Autodesk Inventor part; units mm, degrees
ref_plane "YZ Plane" through (0, 0, 0) normal (1, 0, 0) x (0, 1, 0)
ref_plane "XZ Plane" through (0, 0, 0) normal (0, 1, 0) x (-1, 0, 0)
ref_plane "XY Plane" through (0, 0, 0) normal (0, 0, 1) x (1, 0, 0)
sketch "Sketch1" plane through (0, 0, 0) normal (0, 0, 1) x (1, 0, 0)
  circle A0 centre (8, -7) radius 1.6
  circle A1 centre (-8, 7) radius 1.6
  circle A2 centre (-2.5, 4.7) radius 0.8
  circle A3 centre (2.5001, 4.7) radius 0.8
  line L0 (-11, 10) -> (-11, -10)
  line L1 (-11, -10) -> (11, -10)
  line L2 (11, -10) -> (11, 10)
  line L3 (11, 10) -> (-11, 10)
  line L4 (-11.2, -10.2) -> (-11.2, 10.2)
  line L5 (-11.2, 10.2) -> (11.2, 10.2)
  line L6 (11.2, 10.2) -> (11.2, -10.2)
  line L7 (11.2, -10.2) -> (-11.2, -10.2)
  circle A4 centre (-8, 7) radius 1.4
  circle A5 centre (8, -7) radius 1.4
  line L8 (-12.2, 11.2) -> (-12.2, -11.2)
  line L9 (-12.2, -11.2) -> (12.2, -11.2)
  line L10 (12.2, -11.2) -> (12.2, 11.2)
  line L11 (12.2, 11.2) -> (-12.2, 11.2)
  circle A6 centre (2.54, -5.9) radius 0.4
  circle A7 centre (-2.54, -5.9) radius 0.4
  circle A8 centre (0, -5.9) radius 0.4
  circle A9 centre (3.5, -7.425) radius 0.5
  circle A10 centre (-3.5, -7.425) radius 0.5
  circle A11 centre (0.6, -3.225) radius 0.3
  circle A12 centre (0.6, -4.425) radius 0.3
  circle A13 centre (-0.6, -3.225) radius 0.3
  circle A14 centre (-0.6, -4.425) radius 0.3
  point P0 (0, 0)
  dimension "d6" = 15
  dimension "d7" = 10
  dimension "d0" = 0.2
  dimension "d1" = 0.2
  dimension "d2" = 0.2
  dimension "d3" = 1
extrude "Extrusion1" add sketch "Sketch1" against normal blind 4 contours A4 | A5 | L11 L10 L9 L8
sketch "Sketch2" plane through (0, 0, -4) normal (0, 0, -1) x (-1, 0, 0)
  line L0 (-12.2, -11.2) -> (12.2, -11.2)
  line L1 (12.2, -11.2) -> (12.2, 11.2)
  line L2 (12.2, 11.2) -> (-12.2, 11.2)
  line L3 (-12.2, 11.2) -> (-12.2, -11.2)
  line L4 (11.2, 10.2) -> (11.2, -10.2)
  line L5 (11.2, -10.2) -> (-11.2, -10.2)
  line L6 (-11.2, -10.2) -> (-11.2, 10.2)
  line L7 (-11.2, 10.2) -> (11.2, 10.2)
  line L8 (5, -7.5) -> (-5, -7.5)
  line L9 (-5, -7.5) -> (-5, 7.5)
  line L10 (-5, 7.5) -> (5, 7.5)
  line L11 (5, 7.5) -> (5, -7.5)
  point P0 (0, 0)
  point P1 (-5, 0)
  point P2 (0, -7.5)
  point P3 (0, -11.2)
  dimension "d6" = 15
  dimension "d7" = 10
extrude "Extrusion2" add sketch "Sketch2" against normal blind 0.5 contours L4 L5 L6 L7
sketch "Sketch3" plane through (0, 0, -4) normal (0, 0, -1) x (-1, 0, 0)
  line L0 (5, -7.5) -> (-5, -7.5)
  line L1 (-5, -7.5) -> (-5, 7.5)
  line L2 (-5, 7.5) -> (5, 7.5)
  line L3 (5, 7.5) -> (5, -7.5)
  line L4 (-12.2, -11.2) -> (12.2, -11.2)
  line L5 (12.2, -11.2) -> (12.2, 11.2)
  line L6 (12.2, 11.2) -> (-12.2, 11.2)
  line L7 (-12.2, 11.2) -> (-12.2, -11.2)
  point P0 (0, 0)
extrude "Extrusion3" add sketch "Sketch3" along normal blind 0.5 contours L0 L1 L2 L3 | L7 L6 L5 L4
sketch "Sketch4" plane through (0, 0, 0) normal (0, 0, 1) x (1, 0, 0)
  line L0 (-12.2, -11.2) -> (12.2, -11.2)
  line L1 (12.2, -11.2) -> (12.2, 11.2)
  line L2 (12.2, 11.2) -> (-12.2, 11.2)
  line L3 (-12.2, 11.2) -> (-12.2, -11.2)
  line L4 (-11.2, -10.2) -> (-11.2, 10.2)
  line L5 (-11.2, 10.2) -> (11.2, 10.2)
  line L6 (11.2, 10.2) -> (11.2, -10.2)
  line L7 (11.2, -10.2) -> (-11.2, -10.2)
  line L8 (-11.2, -10.2) -> (-12.2, -10.2)
  line L9 (11.2, -10.2) -> (-11.2, -10.2)
  line L10 (11.2, -10.2) -> (12.2, -10.2)
  point P0 (0, 0)
extrude "Extrusion4" add sketch "Sketch4" along normal blind 5.3 contours L3 L8 L7 L10 L1 L0
sketch "Sketch5" plane through (-12.2, -11.2, -4.5) normal (0, -1, 0) x (1, 0, 0)
  line L0 (23.4, 9.8) -> (0, 9.8)
  circle A0 centre (12.2, 9.8) radius 3.85
  point P0 (12.2, 4.5)
  point P1 (8.35, 9.8)
  point P2 (16.05, 9.8)
  dimension "d14" = 7.7
extrude "Extrusion5" cut sketch "Sketch5" against normal blind 5.3 contours A0 L0 picked at (11.471, 8.7438)
sketch "Sketch6" plane through (0, 0, -4.5) normal (0, 0, -1) x (-1, 0, 0)
  line L0 (12.2, -11.2) -> (12.2, 11.2)
  line L1 (12.2, 11.2) -> (-12.2, 11.2)
  line L2 (-12.2, 11.2) -> (-12.2, -11.2)
  line L3 (-12.2, -11.2) -> (12.2, -11.2)
  line L4 (13.3, 12.3) -> (13.3, -12.3)
  line L5 (13.3, -12.3) -> (-13.3, -12.3)
  line L6 (-13.3, -12.3) -> (-13.3, 12.3)
  line L7 (-13.3, 12.3) -> (13.3, 12.3)
  line L8 (12.2, -11.2) -> (13.3, -11.2)
  line L9 (-12.2, -11.2) -> (-13.3, -11.2)
  point P0 (0, 0)
  dimension "d17" = 1.1
extrude "Extrusion6" add sketch "Sketch6" against normal blind 1 contours L0 L1 L2 L9 L6 L7 L4 L8
sketch "Sketch7" plane through (0, 0, -3.5) normal (0, 0, 1) x (1, 0, 0)
  circle A0 centre (8, -7) radius 1.4
  circle A1 centre (-8, 7) radius 1.4
  line L0 (11.2, 10.2) -> (11.2, -10.2)
  line L1 (-11.2, 10.2) -> (11.2, 10.2)
  line L2 (-11.2, -10.2) -> (-11.2, 10.2)
  line L3 (11.2, -10.2) -> (-11.2, -10.2)
  line L4 (5, -7.5) -> (-5, -7.5)
  line L5 (-5, -7.5) -> (-5, 7.5)
  line L6 (-5, 7.5) -> (5, 7.5)
  line L7 (5, 7.5) -> (5, -7.5)
  point P0 (0, 0)
extrude "Extrusion7" add sketch "Sketch7" along normal blind 1.9
fillet "Fillet1" radius 2 4 edges at (-5, 7.5, -2.8) (5, 7.5, -2.8) (-5, -7.5, -2.8) (5, -7.5, -2.8)
fillet "Fillet2" radius 1 4 edges at (13.3, 12.3, -4) (13.3, -11.2, -4) (-13.3, -11.2, -4) (-13.3, 12.3, -4)
properties part number "buttom cover"
Can you work these out from the model? Positions are in its coordinate system, mm. A direction names the side the tool comes from. Coordinates: 2 decimals unless noted, no trailing zeros. Write each loop counter-clockwise with the first axis right and the second up, starting at its lowest first coordinate (ties: lowest second). Pieces come first, ordered by that corner, then holes. Notation, with made-up numbers: (35.5, 47.5) -> (47.5, 47.5) arc R27 cw to (47.5, 86.5) -> close; hole circle Ø5 at (61, 74.25). An arc over 180 degrees is marked (long way). Answer as CSV lines item,"result".
1) Will these pins go through, and if not, where does the flat tip stop? P1, Ø3, axis at x = 8.5, y = -4, coming from the +Z side; P2, Ø6, axis at x = 9, y = 3, coming from the +Z side; P3, Ø2.5, axis at y = 1, z = 1.5, coming from the +X side; P4, Ø3.5, axis at x = -4.5, z = 0.5, coming from the +Y side.
Check result:
P1,"z = -1.6"
P2,"z = 0"
P3,"through"
P4,"y = 11.2"
2) If we mould it in two halves opening along X, with no side actions, what happens to faces 1 (the flat face through (-12.2, 0, -1)), 2 (the flat face through (0, 0, -4)), 3 (the cylindrical face through (13.015, 11.999, -3.993))? For each: +X half, -X half, draft (parallel to the pull), parting line (faces both ways), or undercut.
Check result:
face 1,"-X half"
face 2,"undercut"
face 3,"+X half"
3) If we section it at A-A on x = 8: Please give me the cut outline in (y, z).
Check result:
outline,"(-11.2, -4.5) -> (12.3, -4.5) -> (12.3, -3.5) -> (11.2, -3.5) -> (11.2, 0) -> (10.2, 0) -> (10.2, -1.6) -> (-5.6, -1.6) -> (-5.6, 0) -> (-8.4, 0) -> (-8.4, -1.6) -> (-10.2, -1.6) -> (-10.2, 5.3) -> (-11.2, 5.3) -> close"
4) If we section it at C-C on z = 3.75: Please give me the cut outline in (x, y), then the cut area to 3 significant figures.
Check result:
outline,"(-12.2, -11.2) -> (-3.52, -11.2) -> (-3.52, -10.2) -> (-12.2, -10.2) -> close; (3.52, -11.2) -> (12.2, -11.2) -> (12.2, -10.2) -> (3.52, -10.2) -> close"
area,"17.4 mm²"
5) If I drill on line 1 (X direction, y = 9.25, z = -1.5); line 2 (Y direction, x = -4.75, z = -0.5); line 3 (Z direction, x = -4, y = 5), over which ranges is the centre line in solid material (lowest first)? Write a range as from..to.
Check result:
line 1,"-12.2..-11.2, 11.2..12.2"
line 2,"-11.2..-10.2, 10.2..11.2"
line 3,"-4.5..-4"
6) On a 3-axis mill with a long thin cutter (end or side, diameter ignored), from which of +Z, -Z, +X, -X, +Y, -Y can I reach the whole of each face in a straight line? I mean faces 4 (the flat face through (0, 7.5, -3)), 5 (the flat face through (0, 11, 0)), 6 (the flat face through (-13.3, 1, -4)), 7 (the flat face through (12.2, 0, -1)). Say none if no direction works.
Check result:
face 4,"+Z"
face 5,"+Z, +X, -X, +Y"
face 6,"+Z, -Z, -X, +Y, -Y"
face 7,"+Z, +X, +Y, -Y"
7) If we section it at D-D on z = 0.5: Please give me the cut outline in (x, y).
Check result:
outline,"(-12.2, -11.2) -> (12.2, -11.2) -> (12.2, -10.2) -> (-12.2, -10.2) -> close"
8) If we section it at B-B on y = -4.75: Please give me the cut outline in (x, z), then the cut area to 3 significant figures.
Check result:
outline,"(-13.3, -4.5) -> (13.3, -4.5) -> (13.3, -3.5) -> (12.2, -3.5) -> (12.2, 0) -> (11.2, 0) -> (11.2, -1.6) -> (5, -1.6) -> (5, -4) -> (-5, -4) -> (-5, -1.6) -> (-11.2, -1.6) -> (-11.2, 0) -> (-12.2, 0) -> (-12.2, -3.5) -> (-13.3, -3.5) -> close"
area,"52.2 mm²"
